The listing builds one solid part. Answer for the finished solid, in the listing's coordinates (mm). A direction names the side the tool comes from. Coordinates: 2 decimals unless noted, no trailing zeros. Order: outer loops, then holes, each group sorted by start corner. A loop starts at its lowest first (then second) coordinate and runs counter-clockwise, first axis right, second up.
```python
from build123d import *

# Parameters (mm, degrees)
SKETCH3_R           = 69.85
BOSS_EXTRUDE1_DEPTH = 6.35
SKETCH4_R           = 64.77
CUT_EXTRUDE1_DEPTH  = 3.81
SKETCH5_W           = 44.45
SKETCH5_H           = 25.4
CUT_EXTRUDE2_DEPTH  = 7.35
FILLET1_R           = 10
BOSS_EXTRUDE2_DEPTH = 31.75
BOSS_EXTRUDE3_DEPTH = 76.2


with BuildPart() as part:
    # Sketch3 → Boss-Extrude1 (new body)
    with BuildSketch(Plane(origin=(0, 0, 0), x_dir=(1, 0, 0), z_dir=(0, 1, 0))):
        Circle(SKETCH3_R)
        with BuildLine():
            Line((-16.448489627, 6.35), (15.301510373, 6.35))
            ThreePointArc((15.301510373, 6.35), (21.651510373, 0), (15.301510373, -6.35))
            Line((15.301510373, -6.35), (-16.448489627, -6.35))
            ThreePointArc((-16.448489627, -6.35), (-22.798489627, 0), (-16.448489627, 6.35))
        make_face(mode=Mode.SUBTRACT)
    extrude(amount=BOSS_EXTRUDE1_DEPTH)

    # Sketch4 → Cut-Extrude1 (cut)
    with BuildSketch(Plane(origin=(0, 6.35, 0), x_dir=(1, 0, 0), z_dir=(0, 1, 0))):
        Circle(SKETCH4_R)
    extrude(amount=-CUT_EXTRUDE1_DEPTH, mode=Mode.SUBTRACT)

    # Sketch5 → Cut-Extrude2 (cut, through all)
    with BuildSketch(Plane(origin=(0, 6.35, 0), x_dir=(1, 0, 0), z_dir=(0, 1, 0))):
        with Locations((0.312165283, -57.905331129)):
            Rectangle(SKETCH5_W, SKETCH5_H)
    extrude(amount=-CUT_EXTRUDE2_DEPTH, mode=Mode.SUBTRACT)

    # Fillet1
    fillet1_edges = [part.edges().sort_by_distance(p)[0] for p in [
        (22.537165283, 1.27, 45.205331129),
        (-21.912834717, 1.27, 45.205331129),
    ]]
    fillet(fillet1_edges, radius=FILLET1_R)

    # Sketch8 → Boss-Extrude2 (add)
    with BuildSketch(Plane.XZ):
        with BuildLine():
            Line((34.258206884, -40.64), (30.448206884, -40.64))
            ThreePointArc((30.448206884, -40.64), (0, -10.191793116), (-30.448206884, -40.64))
            Line((-30.448206884, -40.64), (-34.258206884, -40.64))
            ThreePointArc((-34.258206884, -40.64), (0, -6.381793116), (34.258206884, -40.64))
        make_face()
    extrude(amount=BOSS_EXTRUDE2_DEPTH)

    # Sketch11 → Boss-Extrude3 (add)
    with BuildSketch(Plane(origin=(0, 2.54, 0), x_dir=(1, 0, 0), z_dir=(0, 1, 0))):
        with BuildLine():
            ThreePointArc((-21.912834717, -52.782100893), (-56.087729184, -10.967640358), (-40.18100173, 40.64))
            Line((-40.18100173, 40.64), (-48.791806689, 40.64))
            ThreePointArc((-48.791806689, 40.64), (-61.333240284, -16.446386725), (-21.912834717, -59.599309347))
            Line((-21.912834717, -59.599309347), (-21.912834717, -55.205331129))
            Line((-21.912834717, -55.205331129), (-21.912834717, -52.782100893))
        make_face()
        with BuildLine():
            Line((48.791806689, 40.64), (40.18100173, 40.64))
            ThreePointArc((40.18100173, 40.64), (56.15176968, -10.634907703), (22.537165283, -52.518555588))
            Line((22.537165283, -52.518555588), (22.537165283, -55.205331129))
            Line((22.537165283, -55.205331129), (22.537165283, -59.366035584))
            ThreePointArc((22.537165283, -59.366035584), (61.418705204, -16.124287613), (48.791806689, 40.64))
        make_face()
    extrude(amount=-BOSS_EXTRUDE3_DEPTH)


solid = part.part
```
(1) Find section B-B (y = -46.5). Write down the section's boundary in (x, z), and give its area (3 significant figures).
(2) Each of these flat-tipped pins is pushed along its axis until it touches: pin 1 Ø3 at (x, y) = (31.5, -19) entering from -Z; pin 2 Ø3 at (y, z) = (-53.5, -1.5) entering from +X; pin 3 Ø3 at (x, z) = (53.5, 5.5) entering from -Y; pin 4 Ø3 at (x, y) = (6, -33.5) entering from -Z. Where does it stop, or does it pass through?
(3) Find section C-C (z = 0). Write down the section's boundary in (x, y), and give its area (3 significant figures).
(4) Find section D-D (z = 28). Write down the section's boundary in (x, y).
(5) The mould has two halves that part along Z. Classify faces 4 (the face through (2.426, 3.131, -69.808)), 5 (the face through (-0.75, -15.65, -6.39)), 6 (the face through (45, -36, -40.64)): released by +Z, released by -Z, zero draft, split by the parting line, or undercut.
(6) Consider line 1 (X direction, y = 5.1, z = 0); line 2 (Z direction, x = 0, y = 5.4); line 3 (Y direction, x = 40, z = -19.5). Determine where each line is inside the solid, lowest interval first.
(7) For faces 1 (the face through (-61.55, -36.31, 15.62)), 2 (the face through (56.292, -36.314, 9.865)), 3 (the face through (21.65, 1.25, -0.14)), determine the directions among +Z, -Z, +X, -X, +Y, -Y from which every point of the face is accessible in a straight line to the end or side of a thin tool.
Findings below:
1. outline: (-48.79, -40.64) - (-40.18, -40.64) arc R57.15 cw to (-21.91, 52.78) - (-21.91, 59.6) arc R63.5 ccw to start; (22.54, 52.52) arc R57.15 cw to (40.18, -40.64) - (48.79, -40.64) arc R63.5 ccw to (22.54, 59.37) - close
1. area: 1,480 mm2
2. pin 1: stops at z = -40.64
2. pin 2: stops at x = 63.5
2. pin 3: stops at y = 0
2. pin 4: passes through
3. outline: (-69.85, 0) - (-63.5, 0) - (-63.5, -73.66) - (-57.15, -73.66) - (-57.15, 0) - (-22.8, 0) - (-22.8, 2.54) - (-64.77, 2.54) - (-64.77, 6.35) - (-69.85, 6.35) - close; (21.65, 0) - (57.15, 0) - (57.15, -73.66) - (63.5, -73.66) - (63.5, 0) - (69.85, 0) - (69.85, 6.35) - (64.77, 6.35) - (64.77, 2.54) - (21.65, 2.54) - close
3. area: 1,220 mm2
4. outline: (-63.99, 0) - (-56.99, 0) - (-56.99, -73.66) - (-49.82, -73.66) - (-49.82, 0) - (49.82, 0) - (49.82, -73.66) - (56.99, -73.66) - (56.99, 0) - (63.99, 0) - (63.99, 6.35) - (58.41, 6.35) - (58.41, 2.54) - (-58.41, 2.54) - (-58.41, 6.35) - (-63.99, 6.35) - close
5. face 4: split by the parting line
5. face 5: undercut
5. face 6: released by -Z
6. line 1: x = -69.85 to -64.77, 64.77 to 69.85
6. line 2: z = -69.85 to -64.77
6. line 3: y = 0 to 2.54
7. face 1: -X, -Y
7. face 2: -Y
7. face 3: +Y, -Y
